Work out the finished part from the listing and answer in its coordinate system (mm). A direction names the side the tool comes from. Round coordinates to 2 decimals unless told otherwise and drop trailing zeros. Order: outer loops, then holes, each group sorted by start corner. A loop starts at its lowest first (then second) coordinate and runs counter-clockwise, first axis right, second up. Notation, with made-up numbers: (21.5, 75.5) - (55.5, 75.5) arc R27 cw to (55.5, 95.5) - close; hole circle Ø3 at (-33, 54). An arc over 180 degrees is marked (long way). Put each result on its own line as item: value.
```python
from build123d import *

# Parameters (mm, degrees)
SKETCH_1_R      = 21
EXTRUDE_1_DEPTH = 2
EXTRUDE_3_DEPTH = 1
CHAMFER_1_SIZE  = 0.5


with BuildPart() as part:
    # 草图1 → 凸台-拉伸1 (new body)
    with BuildSketch(Plane.XY):
        Circle(SKETCH_1_R)
    extrude(amount=EXTRUDE_1_DEPTH)

    # 草图3 → 凸台-拉伸3 (add)
    with BuildSketch(Plane(origin=(0, 0, 0), x_dir=(-1, 0, 0), z_dir=(0, 0, -1))):
        with BuildLine():
            Line((0, 22.5), (0, 21))
            ThreePointArc((0, 21), (1.866666667, 20.916872509), (3.718555113, 20.668148148))
            Line((3.718555113, 20.668148148), (3.984166192, 22.144444444))
            ThreePointArc((3.984166192, 22.144444444), (2, 22.410934831), (0, 22.5))
        make_face()
        with BuildLine():
            Line((19.485571585, 11.25), (18.186533479, 10.5))
            ThreePointArc((18.186533479, 10.5), (19.047876294, 8.841855501), (19.758418902, 7.113710881))
            Line((19.758418902, 7.113710881), (21.169734538, 7.621833087))
            ThreePointArc((21.169734538, 7.621833087), (20.408438886, 9.473416608), (19.485571585, 11.25))
        make_face()
        with BuildLine():
            Line((19.485571585, -11.25), (18.186533479, -10.5))
            ThreePointArc((18.186533479, -10.5), (17.181209627, -12.075017008), (16.039863789, -13.554437267))
            Line((16.039863789, -13.554437267), (17.185568345, -14.522611358))
            ThreePointArc((17.185568345, -14.522611358), (18.408438886, -12.937518223), (19.485571585, -11.25))
        make_face()
        with BuildLine():
            Line((0, -22.5), (0, -21))
            ThreePointArc((0, -21), (-1.866666667, -20.916872509), (-3.718555113, -20.668148148))
            Line((-3.718555113, -20.668148148), (-3.984166192, -22.144444444))
            ThreePointArc((-3.984166192, -22.144444444), (-2, -22.410934831), (0, -22.5))
        make_face()
        with BuildLine():
            Line((-19.485571585, -11.25), (-18.186533479, -10.5))
            ThreePointArc((-18.186533479, -10.5), (-19.047876294, -8.841855501), (-19.758418902, -7.113710881))
            Line((-19.758418902, -7.113710881), (-21.169734538, -7.621833087))
            ThreePointArc((-21.169734538, -7.621833087), (-20.408438886, -9.473416608), (-19.485571585, -11.25))
        make_face()
        with BuildLine():
            Line((-19.485571585, 11.25), (-18.186533479, 10.5))
            ThreePointArc((-18.186533479, 10.5), (-17.181209627, 12.075017008), (-16.039863789, 13.554437267))
            Line((-16.039863789, 13.554437267), (-17.185568345, 14.522611358))
            ThreePointArc((-17.185568345, 14.522611358), (-18.408438886, 12.937518223), (-19.485571585, 11.25))
        make_face()
    extrude(amount=-EXTRUDE_3_DEPTH)

    # 倒角1
    chamfer_1_edges = [part.edges().sort_by_distance(p)[0] for p in [
        (-21, 0, 2),
    ]]
    chamfer(chamfer_1_edges, length=CHAMFER_1_SIZE)


solid = part.part
```
1) A cutting plane is placed at A-A on z = 0.55. Write down the section's boundary in (x, y).
Findings below:
outline: (-21.17, 7.62) - (-19.76, 7.11) arc R21 ccw to (-18.19, -10.5) - (-19.49, -11.25) arc R22.5 ccw to (-17.19, -14.52) - (-16.04, -13.55) arc R21 ccw to (0, -21) - (0, -22.5) arc R22.5 ccw to (3.98, -22.14) - (3.72, -20.67) arc R21 ccw to (18.19, -10.5) - (19.49, -11.25) arc R22.5 ccw to (21.17, -7.62) - (19.76, -7.11) arc R21 ccw to (18.19, 10.5) - (19.49, 11.25) arc R22.5 ccw to (17.19, 14.52) - (16.04, 13.55) arc R21 ccw to (0, 21) - (0, 22.5) arc R22.5 ccw to (-3.98, 22.14) - (-3.72, 20.67) arc R21 ccw to (-18.19, 10.5) - (-19.49, 11.25) arc R22.5 ccw to start
2) Straight lines are drawn through the part: L1, parallel to X at y = -10.5, z = 1.1; L2, parallel to X at y = 14, z = 0.9; L3, parallel to X at y = 4.5, z = 0.3. For each, find the intervals that lie inside material, in ascending order. Write a range as from..to.
Findings below:
L1: x = -18.19..18.19
L2: x = -15.65..15.65, 16.57..17.61
L3: x = -20.51..20.51
3) Given pin 1 Ø1 at (x, y) = (18, 12) entering from +Z; pin 2 Ø1.1 at (y, z) = (-22, 0.5) entering from -X; pin 3 Ø0.5 at (y, z) = (22, 0.5) entering from +X, each flat-ended and moving along its own axis, determine where each tip first touches the part or whether it passes through.
Findings below:
pin 1: stops at z = 1
pin 2: stops at x = 0
pin 3: stops at x = 0
4) For faces 1 (the flat face through (18.845, 10.88, 0.493)), 2 (the flat face through (-18.845, 10.88, 0.493)), 3 (the flat face through (0, 21.8, 0.5)), 4 (the flat face through (-3.85, 21.4, 0.49)), determine the directions among +Z, -Z, +X, -X, +Y, -Y from which every point of the face is accessible in a straight line to the end or side of a thin tool.
Findings below:
face 1: +Z, -Z, +X
face 2: +Z, -Z, +Y
face 3: +Z, -Z, +X, +Y
face 4: +Z, -Z, -X
5) For a pull along X with two mould halves and no side action, classify faces 5 (the flat face through (-16.6, -14.03, 0.49)), 6 (the cylindrical face through (-18.392, -12.96, 0.493)), 7 (the flat face through (-2, 22, 1)) as pulls with the +X half, pulls with the -X half, needs draft (parallel to the pull), parting line crosses it, or undercut.
Findings below:
face 5: undercut
face 6: pulls with the -X half
face 7: needs draft
